Input: part model. Units: mm. Frame: model coordinates. A direction names the side the tool comes from. Coordinates: 2 decimals unless noted, no trailing zeros. Order: outer loops, then holes, each group sorted by start corner. A loop starts at its lowest first (then second) coordinate and runs counter-clockwise, first axis right, second up. Notation, with made-up numbers: (29.25, 5) -> (68.25, 5) arc R28 ccw to (68.25, 38) -> close; hole circle Ø6 at (-11, 48). An arc over 180 degrees is marked (long way). Answer as CSV lines item,"result".
from build123d import *
from OCP.BRepFilletAPI import BRepFilletAPI_MakeChamfer

# Parameters (mm, degrees)
BASE_EXTRUDE_DEPTH        = 3.302
BASE_EXTRUDE_DEPTH_BACK   = 3.302
SKETCH3_W                 = 5.08
SKETCH3_H                 = 9.398
CUT_EXTRUDE1_START        = -5.08
CUT_EXTRUDE1_DEPTH        = 5.08
SKETCH5_W                 = 3.5814
SKETCH5_H                 = 2.54
CUT_EXTRUDE2_DEPTH        = 0.127
BOSS_EXTRUDE1_START       = -9.906
SKETCH6_W                 = 0.635
SKETCH6_H                 = 0.635
BOSS_EXTRUDE1_DEPTH       = 13.716
CHAMFER1_SIZE             = 0.508
CHAMFER1_SIZE2            = 0.293293937
CHAMFER1_OF_MIRROR1_SIZE  = 0.508
CHAMFER1_OF_MIRROR1_SIZE2 = 0.293293937


# Read off the part's stored shape, not the designer's step: Cut-Extrude1
with BuildPart() as part:
    # Sketch3 → Base-Extrude (new, two sides: drawn at the far end of the back side and taken through both)
    with BuildSketch(Plane.XY.offset(-BASE_EXTRUDE_DEPTH_BACK)):
        with Locations((1.27, 4.699)):
            Rectangle(SKETCH3_W, SKETCH3_H)
    extrude(amount=BASE_EXTRUDE_DEPTH + BASE_EXTRUDE_DEPTH_BACK)

    # Cut-Extrude1 outline → Cut-Extrude1 (cut)
    with BuildSketch(Plane.ZY.offset(1.27).offset(CUT_EXTRUDE1_START)):
        with BuildLine():
            add(Edge.make_bspline(
                [(-2.286, 3.81), (-1.368133743, 5.298530644), (-0.381370103, 6.898794196), (-1.568138006, 6.86066242), (-1.651, 6.858)],
                knots=[0, 0, 0, 0, 0.930178433, 1, 1, 1, 1], degree=3))
            Line((-2.286, 3.81), (-2.286, 2.54))
            Line((-2.286, 2.54), (3.302, 2.54))
            Line((3.302, 2.54), (3.302, 9.398))
            Line((3.302, 9.398), (-1.651, 9.398))
            Line((-1.651, 9.398), (-1.651, 6.858))
        make_face()
    extrude(amount=CUT_EXTRUDE1_DEPTH, mode=Mode.SUBTRACT)

    # Sketch5 → Cut-Extrude2 (cut, symmetric)
    with BuildSketch(Plane(origin=(1.27, 0, 0), x_dir=(0, 0, -1), z_dir=(1, 0, 0))):
        with Locations((-1.5113, 1.27)):
            Rectangle(SKETCH5_W, SKETCH5_H)
        with BuildLine():
            Line((3.302, 2.54), (3.302, 9.398))
            Line((3.302, 9.398), (1.651, 9.398))
            Line((1.651, 9.398), (1.651, 6.858))
            add(Edge.make_bspline(
                [(2.286, 3.81), (1.368133743, 5.298530644), (0.381370103, 6.898794196), (1.568138006, 6.86066242), (1.651, 6.858)],
                knots=[0, 0, 0, 0, 0.930178433, 1, 1, 1, 1], degree=3))
            Line((2.286, 3.81), (2.286, 2.54))
            Line((2.286, 2.54), (3.302, 2.54))
        make_face()
    extrude(amount=CUT_EXTRUDE2_DEPTH, both=True, mode=Mode.SUBTRACT)

    # Sketch6 → Boss-Extrude1 (add)
    with BuildSketch(Plane.XZ.offset(BOSS_EXTRUDE1_START)):
        Rectangle(SKETCH6_W, SKETCH6_H)
    boss_extrude1 = extrude(amount=BOSS_EXTRUDE1_DEPTH)

    # Chamfer1: one chamfer whose edges measure the first distance from different faces: ONE call of the kernel's chamfer builder (chamfer() names one face for all edges)
    chamfer1_edges_1 = [part.edges().sort_by_distance(p)[0] for p in [
        (-0.3175, 9.906, 0),
    ]]
    chamfer1_side_1 = [part.faces().sort_by_distance(p)[0] for p in [
        (-0.3175, 6.223, 0),
    ]]
    chamfer1_edges_2 = [part.edges().sort_by_distance(p)[0] for p in [
        (0, 9.906, -0.3175),
    ]]
    chamfer1_side_2 = [part.faces().sort_by_distance(p)[0] for p in [
        (0, 6.223, -0.3175),
    ]]
    chamfer1_edges_3 = [part.edges().sort_by_distance(p)[0] for p in [
        (0.3175, 9.906, 0),
    ]]
    chamfer1_side_3 = [part.faces().sort_by_distance(p)[0] for p in [
        (0.3175, 6.223, 0),
    ]]
    chamfer1_edges_4 = [part.edges().sort_by_distance(p)[0] for p in [
        (0, 9.906, 0.3175),
    ]]
    chamfer1_side_4 = [part.faces().sort_by_distance(p)[0] for p in [
        (0, 6.223, 0.3175),
    ]]
    chamfer1 = BRepFilletAPI_MakeChamfer(part.part.solid().wrapped)
    for e in chamfer1_edges_1:
        chamfer1.Add(CHAMFER1_SIZE, CHAMFER1_SIZE2, e.wrapped, chamfer1_side_1[0].wrapped)  # the first distance lies on this face
    for e in chamfer1_edges_2:
        chamfer1.Add(CHAMFER1_SIZE, CHAMFER1_SIZE2, e.wrapped, chamfer1_side_2[0].wrapped)  # the first distance lies on this face
    for e in chamfer1_edges_3:
        chamfer1.Add(CHAMFER1_SIZE, CHAMFER1_SIZE2, e.wrapped, chamfer1_side_3[0].wrapped)  # the first distance lies on this face
    for e in chamfer1_edges_4:
        chamfer1.Add(CHAMFER1_SIZE, CHAMFER1_SIZE2, e.wrapped, chamfer1_side_4[0].wrapped)  # the first distance lies on this face
    add(Compound.cast(chamfer1.Shape()), mode=Mode.REPLACE)

    # Mirror1: Boss-Extrude1 across plane
    add(boss_extrude1.mirror(Plane(origin=(1.27, 0, 0), x_dir=(0, 0, 1), z_dir=(1, 0, 0))))

    # Chamfer1 of Mirror1: one chamfer whose edges measure the first distance from different faces: ONE call of the kernel's chamfer builder (chamfer() names one face for all edges)
    chamfer1_of_mirror1_edges_1 = [part.edges().sort_by_distance(p)[0] for p in [
        (2.8575, 9.906, 0),
    ]]
    chamfer1_of_mirror1_side_1 = [part.faces().sort_by_distance(p)[0] for p in [
        (2.8575, 6.223, 0),
    ]]
    chamfer1_of_mirror1_edges_2 = [part.edges().sort_by_distance(p)[0] for p in [
        (2.54, 9.906, -0.3175),
    ]]
    chamfer1_of_mirror1_side_2 = [part.faces().sort_by_distance(p)[0] for p in [
        (2.54, 6.223, -0.3175),
    ]]
    chamfer1_of_mirror1_edges_3 = [part.edges().sort_by_distance(p)[0] for p in [
        (2.2225, 9.906, 0),
    ]]
    chamfer1_of_mirror1_side_3 = [part.faces().sort_by_distance(p)[0] for p in [
        (2.2225, 6.223, 0),
    ]]
    chamfer1_of_mirror1_edges_4 = [part.edges().sort_by_distance(p)[0] for p in [
        (2.54, 9.906, 0.3175),
    ]]
    chamfer1_of_mirror1_side_4 = [part.faces().sort_by_distance(p)[0] for p in [
        (2.54, 6.223, 0.3175),
    ]]
    chamfer1_of_mirror1 = BRepFilletAPI_MakeChamfer(part.part.solid().wrapped)
    for e in chamfer1_of_mirror1_edges_1:
        chamfer1_of_mirror1.Add(CHAMFER1_OF_MIRROR1_SIZE, CHAMFER1_OF_MIRROR1_SIZE2, e.wrapped, chamfer1_of_mirror1_side_1[0].wrapped)  # the first distance lies on this face
    for e in chamfer1_of_mirror1_edges_2:
        chamfer1_of_mirror1.Add(CHAMFER1_OF_MIRROR1_SIZE, CHAMFER1_OF_MIRROR1_SIZE2, e.wrapped, chamfer1_of_mirror1_side_2[0].wrapped)  # the first distance lies on this face
    for e in chamfer1_of_mirror1_edges_3:
        chamfer1_of_mirror1.Add(CHAMFER1_OF_MIRROR1_SIZE, CHAMFER1_OF_MIRROR1_SIZE2, e.wrapped, chamfer1_of_mirror1_side_3[0].wrapped)  # the first distance lies on this face
    for e in chamfer1_of_mirror1_edges_4:
        chamfer1_of_mirror1.Add(CHAMFER1_OF_MIRROR1_SIZE, CHAMFER1_OF_MIRROR1_SIZE2, e.wrapped, chamfer1_of_mirror1_side_4[0].wrapped)  # the first distance lies on this face
    add(Compound.cast(chamfer1_of_mirror1.Shape()), mode=Mode.REPLACE)


solid = part.part
1. Mould query, pull axis Z, two halves, no side actions, for faces 6 (the face through (2, 0, 0)), 7 (the face through (3, 8, -1.651)), 8 (the face through (0, 1, 3.302)). Classes: released by +Z, released by -Z, zero draft, split by the parting line, or undercut.
Findings:
face 6,"zero draft"
face 7,"undercut"
face 8,"released by +Z"
2. Ray query, line 1 along X through (y, z) = (7.25, -2.5); line 2 along Z through (x, y) = (2.3, 8.25); line 3 along Y through (x, z) = (2.85, 1). Return the intervals inside material, ascending.
Findings:
line 1,"x = -1.27 to 1.14, 1.4 to 3.81"
line 2,"z = -3.3 to -1.65, -0.32 to 0.32"
line 3,"y = 0 to 2.54"
3. Cut plane A-A (z = 1.75). Return the cut outline in (x, y), plus the area to 3 significant figures.
Findings:
outline,"(-1.27, 0) -> (1.14, 0) -> (1.14, 2.54) -> (-1.27, 2.54) -> close; (1.4, 0) -> (3.81, 0) -> (3.81, 2.54) -> (1.4, 2.54) -> close"
area,"12.3 mm2"
4. Cut plane C-C (y = 0.75). Return the cut outline in (x, z).
Findings:
outline,"(-1.27, -3.3) -> (3.81, -3.3) -> (3.81, 3.3) -> (1.4, 3.3) -> (1.4, -0.28) -> (1.14, -0.28) -> (1.14, 3.3) -> (-1.27, 3.3) -> close"
5. Cut plane B-B (y = 3.5). Return the cut outline in (x, z).
Findings:
outline,"(-1.27, -3.3) -> (1.14, -3.3) -> (1.14, -2.29) -> (-1.27, -2.29) -> close; (-0.32, -0.32) -> (0.32, -0.32) -> (0.32, 0.32) -> (-0.32, 0.32) -> close; (1.4, -3.3) -> (3.81, -3.3) -> (3.81, -2.29) -> (1.4, -2.29) -> close; (2.22, -0.32) -> (2.86, -0.32) -> (2.86, 0.32) -> (2.22, 0.32) -> close"
6. Reachability of faces 1 (the face through (3, 3, -2.286)), 2 (the face through (3, 9.398, -2)), 3 (the face through (0, 8, -1.651)), 4 (the face through (1.143, 1, 2)), 5 (the face through (1.143, 6, -2)) from +Z, -Z, +X, -X, +Y, -Y: full face, straight path, thin tool, end or side. Return the list, or none.
Findings:
face 1,"+X, -X"
face 2,"-Z, +X, -X, +Y"
face 3,"+X, -X, +Y"
face 4,"+Z, +Y, -Y"
face 5,"+Z, -Z, +Y"
7. Cut plane D-D (y = 6.5). State how many separate pieces and enclosed holes the cut face has, plus the area to 3 significant figures.
Findings:
separate pieces,"4"
enclosed holes,"0"
area,"11.9 mm2"
8. Contact query for flat-ended pins moving along their axis: pin 1 (0.7 mm diameter, centred on y = 5.5, z = 0, fed in from -X); pin 2 (1.4 mm diameter, centred on x = 2.5, y = 3, fed in from +Z); pin 3 (0.7 mm diameter, centred on x = 2.5, y = -1.5, fed in from +Z); pin 4 (1.3 mm diameter, centred on x = 0.5, z = -2, fed in from +Y). Output: stop coordinate, or through.
Findings:
pin 1,"stops at x = -0.32"
pin 2,"stops at z = 3.3"
pin 3,"stops at z = 0.32"
pin 4,"stops at y = 9.4"
